Input: dimensioned drawing with shaded views. Units: mm. Origin: part minimum x, y, z. A direction names the side the tool comes from. Round coordinates to 2 decimals unless told otherwise and drop trailing zeros. Write each loop counter-clockwise with the first axis right and the second up, starting at its lowest first coordinate (ties: lowest second). Pieces come first, ordered by that corner, then holes. Notation, with made-up numbers: (70, -35.5) -> (92, -35.5) arc R16 cw to (92, -29.5) -> close; hole circle Ø1 at (-27.75, 10). An arc over 180 degrees is marked (long way). Use one line per item in the form item = value. Start each with the question number.
1. Reachability of the marked faces 1 and 2 from +Z, -Z, +X, -X, +Y, -Y: full face, straight path, thin tool, end or side. Return the list, or none.
2. Line query: L1, parallel to Y at x = 42.5, z = 64 (3 decimals). Output: solid intervals per line, ascending.
3. Cut plane B-B, the plane y = 25. Return the cut outline in (x, z) (3 decimals), plus the area to 3 significant figures.
4. Pin query (flat end, axial travel): pin 1 Ø12 at (x, y) = (65.5, 51.5) entering from +Z. Return the tip coordinate at first contact, or that it passes through.
5. Cut plane A-A, the plane z = 76. Return the cut outline in (x, y) (3 decimals), plus the area to 3 significant figures.
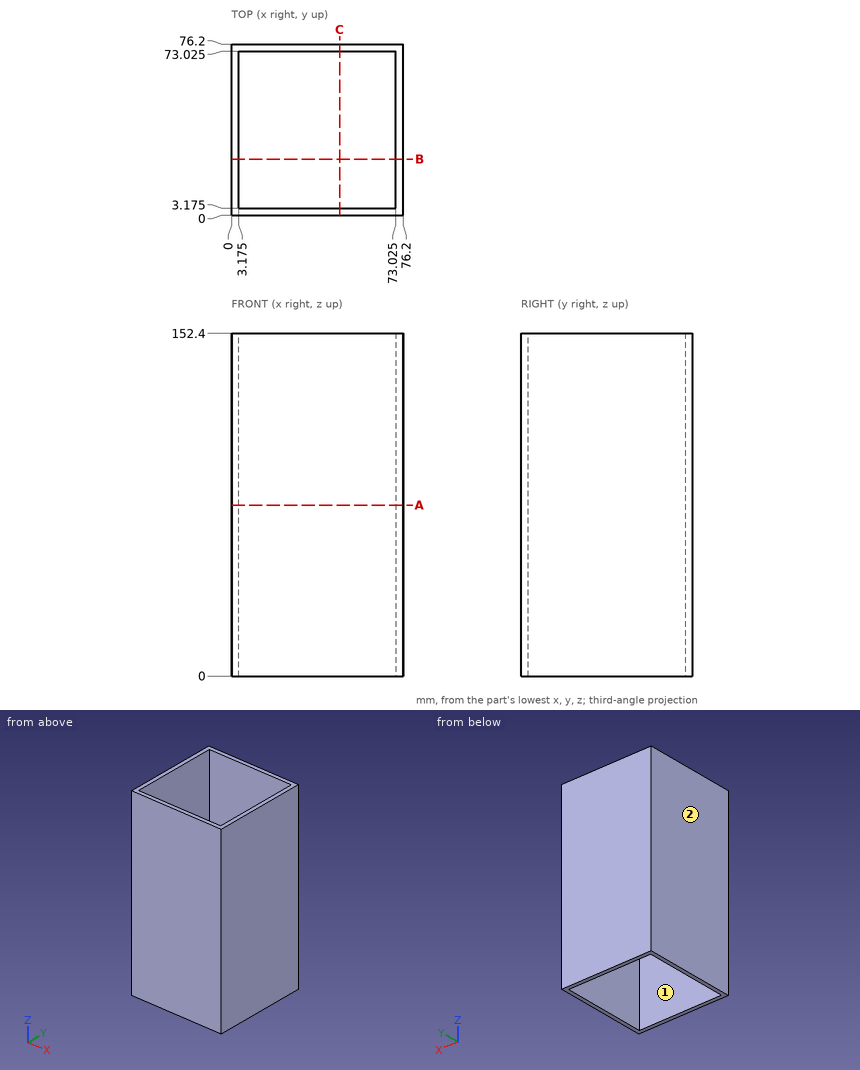
Outcome:
q1.face_1 = +Z, -Z
q1.face_2 = +Z, -Z, -X, +Y, -Y
q2.L1 = 0 to 3.175, 73.025 to 76.2
q3.outline = (0, 0) -> (3.175, 0) -> (3.175, 152.4) -> (0, 152.4) -> close; (73.025, 0) -> (76.2, 0) -> (76.2, 152.4) -> (73.025, 152.4) -> close
q3.area = 968 mm^2
q4.pin_1 = through
q5.outline = (0, 0) -> (76.2, 0) -> (76.2, 76.2) -> (0, 76.2) -> close; hole (3.175, 3.175) -> (73.025, 3.175) -> (73.025, 73.025) -> (3.175, 73.025) -> close
q5.area = 927 mm^2
